The listing builds one solid part. Answer for the finished solid, in the listing's coordinates (mm). Give positions to 0.01 mm unless a question says otherwise; leave off trailing zeros. Order: outer loops, then holes, each group sorted by start corner. A loop starts at its lowest first (then second) coordinate and runs counter-clockwise, first axis right, second up. Notation, with made-up numbers: (25.25, 81) - (54.25, 81) arc R28 ccw to (54.25, 104) - close; hole circle Ø3 at (9.5, 83.25). An arc over 180 degrees is marked (long way). Write each question's results on one line, items separated by ' | '. Start each with the question number.
1. A flat-ended cylindrical pin translates along its axis: pin 1 (5.5 mm diameter, centred on x = 369.5, z = 571, fed in from -Y). Find the tip coordinate at first contact, or state that the pin passes through.
2. Find the intervals of material crossed by L1, parallel to Z at x = 347.5, y = -16; L2, parallel to X at y = -40.5, z = 307.5; L3, parallel to X at y = -16.5, z = 151, in increasing order.
3. Section C-C (y = -12) is taken. Give the vertices of the cut face in (x, z), and give its area (3 significant figures).
4. Section A-A (z = 500) is taken. Give the vertices of the cut face in (x, y).
5. Section B-B (x = 166) is taken. Give the vertices of the cut face in (y, z).
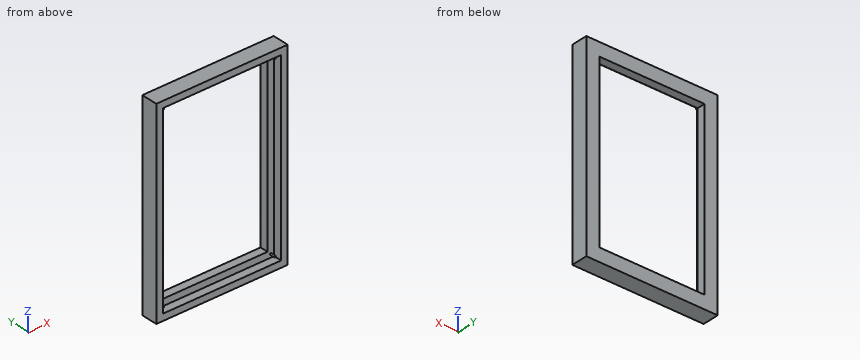
from build123d import *

# Parameters (mm, degrees)
F0_W     = 20
F0_H     = 20
F0_W_2   = 320
F0_H_2   = 520
F1_DEPTH = 50
F0_R     = 2.5
F2_DEPTH = 25
F3_DEPTH = 40


with BuildPart() as f1:
    # F0 (on Front) → F1 (new body)
    with BuildSketch(Plane.XZ):
        with Locations((390, 10)):
            Rectangle(F0_W, F0_H)
        with Locations((370, 10)):
            Rectangle(F0_W, F0_H)
        with Locations((200, 10)):
            Rectangle(F0_W_2, F0_H)
        with Locations((390, 300)):
            Rectangle(F0_W, F0_H_2)
        with Locations((390, 30)):
            Rectangle(F0_W, F0_H)
        with Locations((30, 10)):
            Rectangle(F0_W, F0_H)
        with Locations((10, 10)):
            Rectangle(F0_W, F0_H)
        with Locations((10, 30)):
            Rectangle(F0_W, F0_H)
        with Locations((10, 300)):
            Rectangle(F0_W, F0_H_2)
        with Locations((390, 570)):
            Rectangle(F0_W, F0_H)
        with Locations((390, 590)):
            Rectangle(F0_W, F0_H)
        with Locations((370, 590)):
            Rectangle(F0_W, F0_H)
        with Locations((200, 590)):
            Rectangle(F0_W_2, F0_H)
        with Locations((30, 590)):
            Rectangle(F0_W, F0_H)
        with Locations((10, 590)):
            Rectangle(F0_W, F0_H)
        with Locations((10, 570)):
            Rectangle(F0_W, F0_H)
    extrude(amount=F1_DEPTH)

    # F0 (on Front) → F2 (join)
    with BuildSketch(Plane.XZ):
        with Locations((370, 570)):
            Rectangle(F0_W, F0_H)
        with Locations((370, 570)):
            Circle(F0_R, mode=Mode.SUBTRACT)
        with Locations((200, 570)):
            Rectangle(F0_W_2, F0_H)
        with Locations((370, 300)):
            Rectangle(F0_W, F0_H_2)
        with Locations((30, 570)):
            Rectangle(F0_W, F0_H)
        with Locations((30, 570)):
            Circle(F0_R, mode=Mode.SUBTRACT)
        with Locations((30, 300)):
            Rectangle(F0_W, F0_H_2)
        with Locations((30, 30)):
            Rectangle(F0_W, F0_H)
        with Locations((30, 30)):
            Circle(F0_R, mode=Mode.SUBTRACT)
        with Locations((200, 30)):
            Rectangle(F0_W_2, F0_H)
        with Locations((370, 30)):
            Rectangle(F0_W, F0_H)
        with Locations((370, 30)):
            Circle(F0_R, mode=Mode.SUBTRACT)
    extrude(amount=F2_DEPTH)

    # F0 (on Front) → F3 (join)
    with BuildSketch(Plane.XZ):
        with Locations((370, 30)):
            Circle(F0_R)
        with Locations((30, 30)):
            Circle(F0_R)
        with Locations((30, 570)):
            Circle(F0_R)
        with Locations((370, 570)):
            Circle(F0_R)
    extrude(amount=F3_DEPTH)


solid = f1.part
Reported:
1) pin 1: y = -40
2) L1: 0 to 40, 560 to 600 | L2: 0 to 20, 380 to 400 | L3: 0 to 40, 360 to 400
3) outline: (0, 0) - (400, 0) - (400, 600) - (0, 600) - close; hole (40, 40) - (360, 40) - (360, 560) - (40, 560) - close | area: 73,600 mm²
4) outline: (0, -50) - (20, -50) - (20, -25) - (40, -25) - (40, 0) - (0, 0) - close; (360, -25) - (380, -25) - (380, -50) - (400, -50) - (400, 0) - (360, 0) - close
5) outline: (-50, 0) - (0, 0) - (0, 40) - (-25, 40) - (-25, 20) - (-50, 20) - close; (-50, 580) - (-25, 580) - (-25, 560) - (0, 560) - (0, 600) - (-50, 600) - close
